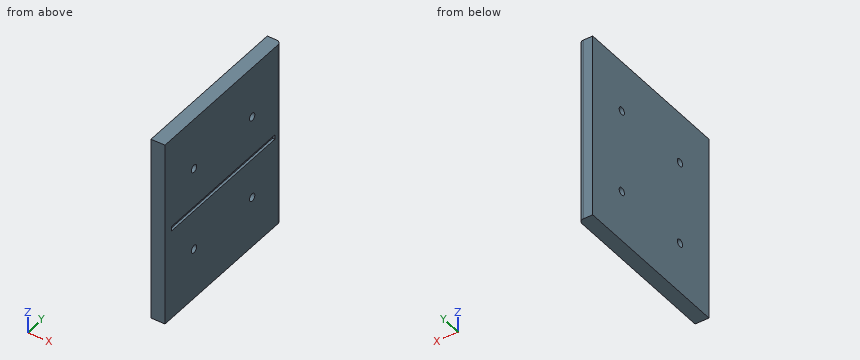
Autodesk Inventor part; units mm, degrees
ref_plane "YZ Plane" through (0, 0, 0) normal (1, 0, 0) x (0, 1, 0)
ref_plane "XZ Plane" through (0, 0, 0) normal (0, 1, 0) x (-1, 0, 0)
ref_plane "XY Plane" through (0, 0, 0) normal (0, 0, 1) x (1, 0, 0)
sketch "Sketch1" plane through (0, 0, 0) normal (1, 0, 0) x (0, 1, 0)
  line L0 (0, 0) -> (-127, 0)
  line L1 (-127, 0) -> (-127, 127)
  line L2 (-127, 127) -> (0, 127)
  line L3 (0, 127) -> (0, 0)
  line L4 (-19.05, 65.0875) -> (-120.65, 65.0875)
  line L5 (-120.65, 65.0875) -> (-120.65, 61.9125)
  line L6 (-120.65, 61.9125) -> (-19.05, 61.9125)
  line L7 (-19.05, 61.9125) -> (-19.05, 65.0875)
  line L8 (0, 47.625) -> (-12.7, 47.625)
  line L9 (-12.7, 47.625) -> (-12.7, 79.375)
  line L10 (-12.7, 79.375) -> (0, 79.375)
  line L11 (0, 79.375) -> (0, 47.625)
  line L12 (-12.7, 47.625) -> (-12.7, 0)
  line L13 (-12.7, 79.375) -> (-12.7, 127)
  dimension "d0" = 127
  dimension "d1" = 127
  dimension "d2" = 6.35
  dimension "d4" = 3.175
  dimension "d5" = 61.9125
  dimension "d25" = 12.7
  dimension "d26" = 31.75
  dimension "d27" = 47.625
  dimension "d28" = 6.35
extrude "Extrusion1" add sketch "Sketch1" along normal blind 9.525 contours L0 L1 L2 L13 L9 L12
extrude "Extrusion2" add sketch "Sketch1" along normal blind 7.9375 contours L7 L6 L5 L4
sketch "Sketch3" plane through (0, 0, 0) normal (-1, 0, 0) x (0, 0, 1)
  circle A0 centre (34.925, -41.275) radius 2.5797
  line L0 (0, -127) -> (0, -12.7)
  line L1 (0, -12.7) -> (0, 0)
  line L2 (0, 0) -> (20.4302, 0)
  line L3 (20.4302, 0) -> (0, -12.7)
  circle A1 centre (34.925, -98.425) radius 2.5797
  circle A2 centre (92.075, -41.275) radius 2.5797
  circle A3 centre (92.075, -98.425) radius 2.5797
  line L4 (0, -12.7) -> (127, -12.7)
  dimension "d31" = 57.15
  dimension "d34" = 57.15
  dimension "d37" = 34.925
  dimension "d38" = 28.575
  dimension "d39" = 5.1594
extrude "Extrusion4" cut sketch "Sketch3" against normal through all contours A0 | A1 | A2 | A3
fillet "Fillet5" radius 3.175 1 edges at (9.525, -12.7, 63.5)
equation "\"d5\" = -0.5 * d4 + 0.5 * d1"
equation "\"d27\" = -0.5 * d26 + 0.5 * d1"
equation "\"d28\" = d2"
properties part number "Gripper plate"
Geometry: final body of the model. Coordinates: model frame, mm. Round coordinates to 2 decimals unless told otherwise and drop trailing zeros. Order: outer loops, then holes, each group sorted by start corner. A loop starts at its lowest first (then second) coordinate and runs counter-clockwise, first axis right, second up. Notation, with made-up numbers: (-17.5, 2.5) - (12.5, 2.5) arc R29 ccw to (12.5, 29.5) - close; hole circle Ø6 at (-10.5, 61.5). An arc over 180 degrees is marked (long way). Use CSV: the item, a comma, the result in double quotes. Start each with the question number.
Q1. Material intervals for line 1 along Z through (x, y) = (8.5, -109); line 2 along Y through (x, z) = (5.75, 93.5); line 3 along Y through (x, z) = (6.75, 55.5), sorted ascending. Write a range as from..to.
Q2. Section query A-A (z = 36). Return loops of the section in (x, y) (3 decimals).
Q3. First-contact query: pin 1 (3.5 mm diameter, centred on y = -46, z = 63, fed in from +X) (3 decimals); pin 2 (4 mm diameter, centred on y = -41.275, z = 92.075, fed in from -X); pin 3 (1.7 mm diameter, centred on x = 8.5, z = 63.5, fed in from +Y). Flat tips, straight axial feed; report the tip coordinate or a pass-through.
Result set:
1,line 1,"z = 0..61.91, 65.09..127"
1,line 2,"y = -127..-100.58, -96.27..-43.43, -39.12..-12.7"
1,line 3,"y = -127..-12.73"
2,outline,"(0, -127) - (9.525, -127) - (9.525, -100.77) - (0, -100.77) - close; (0, -96.08) - (9.525, -96.08) - (9.525, -43.62) - (0, -43.62) - close; (0, -38.93) - (9.525, -38.93) - (9.525, -15.875) arc R3.175 ccw to (6.35, -12.7) - (0, -12.7) - close"
3,pin 1,"stops at x = 9.525"
3,pin 2,"passes through"
3,pin 3,"stops at y = -12.98"
